```python
from build123d import *

# Parameters (mm, degrees)
F0_W     = 60
F0_H     = 40
F1_DEPTH = 40
F3_DEPTH = 30


with BuildPart() as f1:
    # F0 (on Front) → F1 (new body)
    with BuildSketch(Plane.XZ):
        with Locations((0.457271, -20)):
            Rectangle(F0_W, F0_H)
    extrude(amount=F1_DEPTH)

    # F2 (on face) → F3 (cut)
    with BuildSketch(Plane.XY):
        Polygon((9.295005, 0), (-10.704995, 0), (-16.427813, -40), (19.328658, -40), align=None)
    extrude(amount=-F3_DEPTH, mode=Mode.SUBTRACT)


solid = f1.part
```
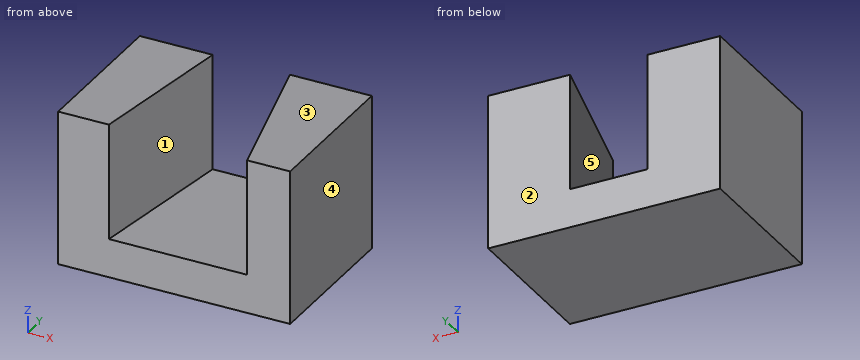
CAD build for the part. Positions are in the model's coordinates, mm. Face numbers are marked on the shaded views. A direction names the side the tool comes from. Round coordinates to 2 decimals unless told otherwise and drop trailing zeros. Order: outer loops, then holes, each group sorted by start corner. A loop starts at its lowest first (then second) coordinate and runs counter-clockwise, first axis right, second up. Notation, with made-up numbers: (-14, -10.5) - (43, -10.5) arc R29 cw to (43, 12.5) - close; hole circle Ø2 at (-30.75, 66). An arc over 180 degrees is marked (long way). Use CSV: the item, a comma, the result in double quotes. Start each with the question number.
1) Saw through at D-D (y = -34.5). List the corners of the cut face in (x, z), and give its area (3 significant figures).
2) Saw through at B-B (y = -22.5). List the corners of the cut face in (x, z), and give its area (3 significant figures).
3) Wall check: L1, parallel to Z at x = 5.5, y = -6.5; L2, parallel to X at y = -3.5, z = -18.5; L3, parallel to X at y = -35.5, z = -15.5. Give the ranges that are in metal, low to high. Write a range as [from, to].
4) Saw through at A-A (z = -24). List the corners of the cut face in (x, y) (3 decimals).
5) Saw through at C-C (x = 15). List the corners of the cut face in (y, z), and give its area (3 significant figures).
6) Two-plate mould, pull along X, no slides. Class the marked faces 3, 4 and 5: pulls with the +X half, pulls with the -X half, needs draft (parallel to the pull), parting line crosses it, or undercut.
7) Tool access for the marked faces 1 and 2: list every direction of +Z, -Z, +X, -X, +Y, -Y with a clear straight run to the whole face (end or side of a thin tool).
Values follow:
1,outline,"(-29.54, -40) - (30.46, -40) - (30.46, 0) - (17.95, 0) - (17.95, -30) - (-15.64, -30) - (-15.64, 0) - (-29.54, 0) - close"
1,area,"1,390 mm2"
2,outline,"(-29.54, -40) - (30.46, -40) - (30.46, 0) - (14.94, 0) - (14.94, -30) - (-13.92, -30) - (-13.92, 0) - (-29.54, 0) - close"
2,area,"1,530 mm2"
3,L1,"z = [-40, -30]"
3,L2,"x = [-29.54, -11.21], [10.17, 30.46]"
3,L3,"x = [-29.54, -15.78], [18.2, 30.46]"
4,outline,"(-29.543, -40) - (-16.428, -40) - (-10.705, 0) - (-29.543, 0) - close; (9.295, 0) - (19.329, -40) - (30.457, -40) - (30.457, 0) - close"
5,outline,"(-40, -40) - (0, -40) - (0, 0) - (-22.74, 0) - (-22.74, -30) - (-40, -30) - close"
5,area,"1,080 mm2"
6,face 3,"needs draft"
6,face 4,"pulls with the +X half"
6,face 5,"undercut"
7,face 1,"+Z, -Y"
7,face 2,"+Z, -Z, +X, -X, +Y"
